from build123d import *

# Parameters (mm, degrees)
SKETCH1_R                 = 3.5
SKETCH1_R_2               = 15
BOSS_EXTRUDE1_DEPTH       = 10
BOSS_EXTRUDE2_DEPTH       = 3.5
SKETCH2_R                 = 21
CUT_EXTRUDE1_DEPTH        = 9
F_1_0MM_DOWEL_HOLE1_D     = 7
F_1_0MM_DOWEL_HOLE1_DEPTH = 5
SKETCH6_R                 = 4.5
CUT_EXTRUDE2_DEPTH        = 20
M6_TAPPED_HOLE1_D         = 5
M6_TAPPED_HOLE1_DEPTH     = 15
M6_TAPPED_HOLE2_D         = 5
M6_TAPPED_HOLE2_DEPTH     = 15


with BuildPart() as part:
    # Sketch1 → Boss-Extrude1 (new, symmetric)
    with BuildSketch(Plane(origin=(0, 0, 0), x_dir=(1, 0, 0), z_dir=(0, 1, 0))):
        with BuildLine():
            Line((-85, 20), (-85, 0))
            Line((-85, 0), (85, 0))
            Line((85, 0), (85, 20))
            Line((85, 20), (68, 20))
            ThreePointArc((68, 20), (65.878679656, 20.878679656), (65, 23))
            Line((65, 23), (65, 187))
            Line((65, 187), (42.75, 187))
            Line((42.75, 187), (42.75, 100))
            ThreePointArc((42.75, 100), (41.871320344, 97.878679656), (39.75, 97))
            Line((39.75, 97), (32.75, 97))
            Line((32.75, 97), (-32.75, 97))
            Line((-32.75, 97), (-39.75, 97))
            ThreePointArc((-39.75, 97), (-41.871320344, 97.878679656), (-42.75, 100))
            Line((-42.75, 100), (-42.75, 187))
            Line((-42.75, 187), (-65, 187))
            Line((-65, 187), (-65, 23))
            ThreePointArc((-65, 23), (-65.878679656, 20.878679656), (-68, 20))
            Line((-68, 20), (-85, 20))
        make_face()
        with Locations(Location((-35, 22.5, 0), (0, 0, 270))):
            Circle(SKETCH1_R, mode=Mode.SUBTRACT)
        with Locations(Location((35, 22.5, 0), (0, 0, 270))):
            Circle(SKETCH1_R, mode=Mode.SUBTRACT)
        with Locations(Location((0, 65, 0), (0, 0, 270))):
            Circle(SKETCH1_R_2, mode=Mode.SUBTRACT)
    extrude(amount=BOSS_EXTRUDE1_DEPTH, both=True)

    # Sketch1_4 → Boss-Extrude2 (add, symmetric)
    with BuildSketch(Plane(origin=(0, 0, 0), x_dir=(1, 0, 0), z_dir=(0, 1, 0))):
        with BuildLine():
            Line((-35.75, 187), (-42.75, 187))
            Line((-42.75, 187), (-42.75, 100))
            ThreePointArc((-42.75, 100), (-41.871320344, 97.878679656), (-39.75, 97))
            Line((-39.75, 97), (-32.75, 97))
            ThreePointArc((-32.75, 97), (-34.871320344, 97.878679656), (-35.75, 100))
            Line((-35.75, 100), (-35.75, 187))
        make_face()
        with BuildLine():
            Line((35.75, 187), (35.75, 100))
            ThreePointArc((35.75, 100), (34.871320344, 97.878679656), (32.75, 97))
            Line((32.75, 97), (39.75, 97))
            ThreePointArc((39.75, 97), (41.871320344, 97.878679656), (42.75, 100))
            Line((42.75, 100), (42.75, 187))
            Line((42.75, 187), (35.75, 187))
        make_face()
    extrude(amount=BOSS_EXTRUDE2_DEPTH, both=True)

    # Sketch2 → Cut-Extrude1 (cut)
    with BuildSketch(Plane.XZ.offset(10)):
        with Locations(Location((0, -65, 0), (0, 0, 270))):
            Circle(SKETCH2_R)
    extrude(amount=-CUT_EXTRUDE1_DEPTH, mode=Mode.SUBTRACT)

    # 1.0mm Dowel Hole1
    with Locations(Plane(origin=(0, 0, -97), x_dir=(-1, 0, 0), z_dir=(0, 0, -1))):
        with Locations((-25, 0), (25, 0)):
            Hole(F_1_0MM_DOWEL_HOLE1_D / 2, depth=F_1_0MM_DOWEL_HOLE1_DEPTH)

    # Sketch6 → Cut-Extrude2 (cut)
    with BuildSketch(Plane.XY):
        with Locations((77, 0)):
            Circle(SKETCH6_R)
        with Locations((-77, 0)):
            Circle(SKETCH6_R)
    extrude(amount=-CUT_EXTRUDE2_DEPTH, mode=Mode.SUBTRACT)

    # M6 Tapped Hole1
    with Locations(Plane(origin=(0, 0, -187), x_dir=(-1, 0, 0), z_dir=(0, 0, -1))):
        with Locations((55, 0)):
            Hole(M6_TAPPED_HOLE1_D / 2, depth=M6_TAPPED_HOLE1_DEPTH)

    # M6 Tapped Hole2
    with Locations(Plane(origin=(0, 0, -187), x_dir=(-1, 0, 0), z_dir=(0, 0, -1))):
        with Locations((-55, 0)):
            Hole(M6_TAPPED_HOLE2_D / 2, depth=M6_TAPPED_HOLE2_DEPTH)


solid = part.part
Could you check a few things on this model? Use its own coordinates, in mm. A direction names the side the tool comes from. Give positions to 0.01 mm unless a question says otherwise; leave off trailing zeros. Order: outer loops, then holes, each group sorted by start corner. A loop starts at its lowest first (then second) coordinate and runs counter-clockwise, first axis right, second up. Notation, with made-up numbers: (-23, 38.5) - (25, 38.5) arc R20 cw to (25, 67.5) - close; hole circle Ø2 at (-13.5, 28.25). An arc over 180 degrees is marked (long way). Return JSON: item names as keys, results as strings. Group by question number.
Q1. Thinking about a two-plate mould opening in X: for faces 1 (the face through (-85, 0, -10)), 2 (the face through (-20, -10, -74)), 3 (the face through (38.47, -0.14, -22.96)), which applies, pulls with the +X half, pulls with the -X half, needs draft (parallel to the pull), parting line crosses it, or undercut?
Q2. Suppose I cut it at D-D, the plane x = 0. Please give me the cut outline in (y, z), and give its area (3 significant figures).
Q3. Which directions (+Z, -Z, +X, -X, +Y, -Y) give clear straight access to the entire face, cutting with the end or side of a thin tool? Please do faces 4 (the face through (-42.75, -7, -143)), 5 (the face through (-52.69, -0.96, -179.4)), 6 (the face through (0.92, -5.56, -44.02)), 7 (the face through (-35.75, 0, -143)).
Q4. Please list where these lines run through material, in increasing order: line 1 along X through (y, z) = (0, -22.5); line 2 along Z through (x, y) = (0, 5); line 3 along X through (y, z) = (-0.5, -123.5). Write a range as [from, to].
Q5. Will these pins go through, and if not, where does the flat tip stop? pin 1 Ø1.5 at (y, z) = (-4, -151) entering from -X; pin 2 Ø7 at (y, z) = (-7, -129) entering from +X; pin 3 Ø2 at (x, y) = (-25.5, 1.5) entering from -Z.
Q6. Suppose I cut it at B-B, the plane z = -65. Please give me the cut outline in (x, y), and give its area (3 significant figures).
Q7. Suppose I cut it at A-A, the plane x = 77. Please give me the cut outline in (y, z).
Q8. Suppose I cut it at C-C, the plane y = -7.25. Please give me the cut outline in (x, z), and give its area (3 significant figures).
Resolved:
{
 "1": {"face 1": "pulls with the -X half", "face 2": "needs draft", "face 3": "undercut"},
 "2": {"outline": "(-10, -97) - (10, -97) - (10, -80) - (-1, -80) - (-1, -86) - (-10, -86) - close; (-10, -44) - (-1, -44) - (-1, -50) - (10, -50) - (10, 0) - (-10, 0) - close", "area": "1,230 mm2"},
 "3": {"face 4": "-Z, -Y", "face 5": "-Z", "face 6": "-Y", "face 7": "-Z, +Y, -Y"},
 "4": {"line 1": "x = [-65.04, -38.5], [-31.5, 31.5], [38.5, 65.04]", "line 2": "z = [-97, -80], [-50, 0]", "line 3": "x = [-65, -35.75], [35.75, 65]"},
 "5": {"pin 1": "stops at x = -65", "pin 2": "stops at x = 65", "pin 3": "stops at z = -92"},
 "6": {"outline": "(-65, -10) - (-21, -10) - (-21, -1) - (-15, -1) - (-15, 10) - (-65, 10) - close; (15, -1) - (21, -1) - (21, -10) - (65, -10) - (65, 10) - (15, 10) - close", "area": "1,890 mm2"},
 "7": {"outline": "(-10, -20) - (-4.5, -20) - (-4.5, 0) - (-10, 0) - close; (4.5, -20) - (10, -20) - (10, 0) - (4.5, 0) - close"},
 "8": {"outline": "(-85, -20) - (-68, -20) arc R3 cw to (-65, -23) - (-65, -187) - (-42.75, -187) - (-42.75, -100) arc R3 cw to (-39.75, -97) - (39.75, -97) arc R3 cw to (42.75, -100) - (42.75, -187) - (65, -187) - (65, -23) arc R3 cw to (68, -20) - (85, -20) - (85, 0) - (-85, 0) - close; hole circle Ø7 at (-35, -22.5); hole circle Ø42 at (0, -65); hole circle Ø7 at (35, -22.5)", "area": "16,000 mm2"}
}
